Drawing for the job (mm, zero at the part's lowest x, y, z). Round coordinates to 2 decimals unless told otherwise and drop trailing zeros. Loops run counter-clockwise (first coordinate to the right, second up) from the corner with the lowest first, then second, coordinate; pieces in that order, holes last.
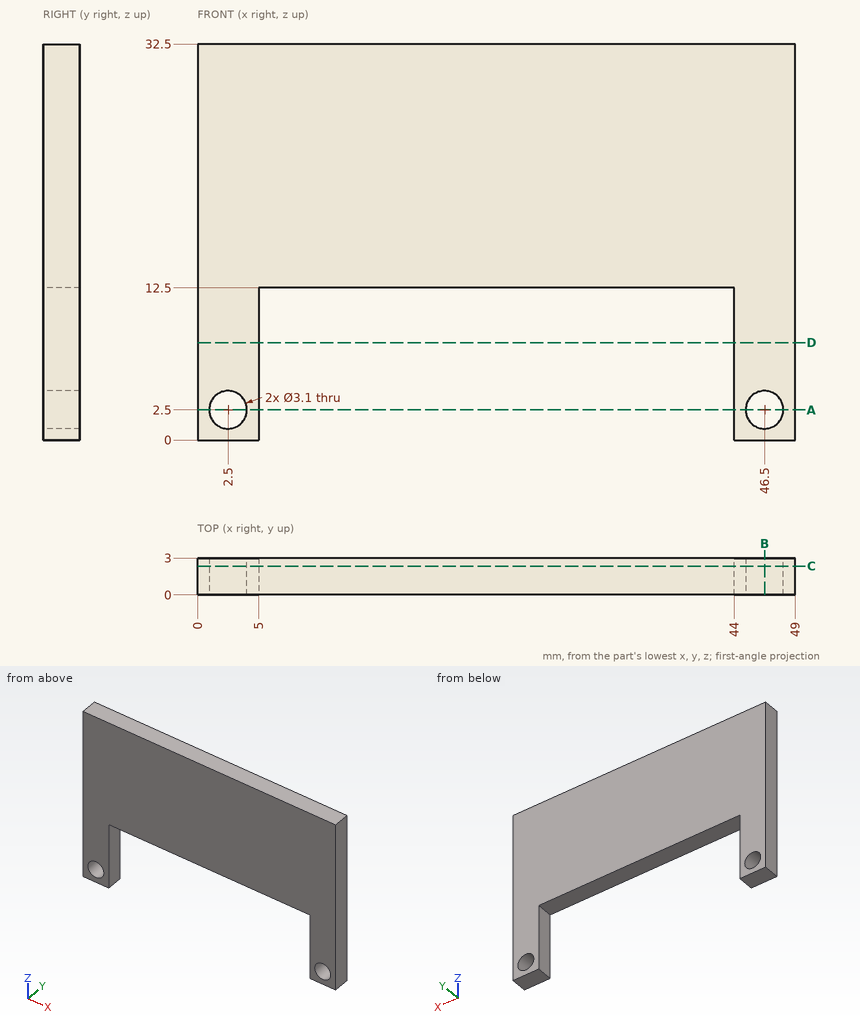
Q1. Slice it at B-B on x = 46.5. Give the cut face in (y, z), plus the area to 3 significant figures.
Q2. Slice it at D-D on z = 8. Give the cut face in (x, y).
Q3. Slice it at C-C on y = 2.35. Give the cut face in (x, z).
Q4. Probe line 1 (Z direction, x = 2.5, y = 0.8); line 2 (Z direction, x = 6, y = 2.7); line 3 (X direction, y = 1.15, z = 11). List the from-to ranges inside material, lowest first.
Q5. Flat gauge pin, fed straight in: P1, Ø3, axis at x = 2.5, z = 2.5, coming from the -Y side (3 decimals). Where does the tip first touch, or does it go through?
Q6. Slice it at A-A on z = 2.5. Give the cut face in (x, y).
Reply:
1. outline: (0, 0) - (3, 0) - (3, 0.95) - (0, 0.95) - close; (0, 4.05) - (3, 4.05) - (3, 32.5) - (0, 32.5) - close
1. area: 88.2 mm2
2. outline: (0, 0) - (5, 0) - (5, 3) - (0, 3) - close; (44, 0) - (49, 0) - (49, 3) - (44, 3) - close
3. outline: (0, 0) - (5, 0) - (5, 12.5) - (44, 12.5) - (44, 0) - (49, 0) - (49, 32.5) - (0, 32.5) - close; hole circle Ø3.1 at (2.5, 2.5); hole circle Ø3.1 at (46.5, 2.5)
4. line 1: z = 0 to 0.95, 4.05 to 32.5
4. line 2: z = 12.5 to 32.5
4. line 3: x = 0 to 5, 44 to 49
5. P1: passes through
6. outline: (0, 0) - (0.95, 0) - (0.95, 3) - (0, 3) - close; (4.05, 0) - (5, 0) - (5, 3) - (4.05, 3) - close; (44, 0) - (44.95, 0) - (44.95, 3) - (44, 3) - close; (48.05, 0) - (49, 0) - (49, 3) - (48.05, 3) - close
